Here's how the part is built. I have some questions about the finished solid (model axes, mm). A direction names the side the tool comes from. Coordinates: 2 decimals unless noted, no trailing zeros. Loops run counter-clockwise (first coordinate to the right, second up) from the corner with the lowest first, then second, coordinate; pieces in that order, holes last. Notation, with made-up numbers: (18, 41) -> (24, 41) arc R23 cw to (24, 58) -> close; hole circle Ø9 at (59.5, -37.75). An arc over 180 degrees is marked (long way). Answer as a JSON object with one key per item and string values. Group by question number.
1) I want a section at C-C (x = -20.5). Write out the boundary of the cut face in (y, z) (3 decimals), then the cut area to 3 significant figures.
2) I want a section at A-A (x = 0). Count the separate pieces of the cut face and the enclosed holes in it, then the cut area to 3 significant figures.
3) I need wall thicknesses on probe 1 along Y at (x, z) = (7.5, 11) (3 decimals); probe 2 along X at (y, z) = (-8, 16.5) (3 decimals); probe 3 along Z at (x, y) = (-11, -1.5). Which ranges of each line are inside material? Lowest first, please. Write a range as [from, to].
4) Which directions (+Z, -Z, +X, -X, +Y, -Y) give clear straight access to the entire face, cutting with the end or side of a thin tool? Please do faces 5 (the flat face through (-7, 6.096, 10)), 6 (the cylindrical face through (3.714, 8.478, 12.804)), 7 (the flat face through (-1, -6.223, 83)).
5) I'm going to push flat-ended pins straight in: pin 1 (4 mm diameter, centred on x = 5.14, z = 14.67, fed in from +Y); pin 2 (6 mm diameter, centred on x = -6.5, y = 0, fed in from -Z); pin 3 (1 mm diameter, centred on y = 5, z = 20.5, fed in from -X); pin 4 (4 mm diameter, centred on y = -4.5, z = 31, fed in from -X). Where does each tip first touch, or does it pass through?
6) If we mould it in two halves opening along X, with no side actions, what happens to faces 1 (the cylindrical face through (0.103, 8.541, 77.028)), 2 (the cylindrical face through (0.87, -8.54, 88.86)), 3 (the flat face through (9.525, 0, 39)), 4 (the flat face through (-7, -6.096, 10))? For each: +X half, -X half, draft (parallel to the pull), parting line (faces both ways), or undercut.
7) I want a section at D-D (y = 0). Write out the boundary of the cut face in (x, z) (3 decimals), then the cut area to 3 significant figures.
8) I want a section at B-B (z = 70). Write out the boundary of the cut face in (x, y) (3 decimals), then the cut area to 3 significant figures.
```python
from build123d import *

# Parameters (mm, degrees)
SKETCH1_W                    = 19.05
SKETCH1_H                    = 21.59
BOSS_EXTRUDE1_DEPTH          = 88.9
CUT_EXTRUDE_THIN1_DEPTH      = 92.978604713
CUT_EXTRUDE_THIN1_DEPTH_BACK = 88.9
SKETCH4_R                    = 2.3495
CUT_EXTRUDE1_DEPTH           = 92.978604713
BOSS_EXTRUDE2_START          = -21.59
SKETCH5_R                    = 2.3495
BOSS_EXTRUDE2_DEPTH          = 21.59
SKETCH6_W                    = 38.1
SKETCH6_H                    = 12.192
CUT_EXTRUDE2_DEPTH           = 96.446647008


with BuildPart() as part:
    # Sketch1 → Boss-Extrude1 (new body)
    with BuildSketch(Plane.XY):
        Rectangle(SKETCH1_W, SKETCH1_H)
    extrude(amount=BOSS_EXTRUDE1_DEPTH)

    # Sketch3 → Cut-Extrude-Thin1 (cut, two sides: drawn at the far end of the back side and taken through both)
    with BuildSketch(Plane(origin=(0, 10.795, 0), x_dir=(1, 0, 0), z_dir=(0, 1, 0)).offset(-CUT_EXTRUDE_THIN1_DEPTH_BACK)):
        with BuildLine():
            ThreePointArc((-9.525, -79.375), (0, -88.9), (9.525, -79.375))
            Line((9.525, -79.375), (34.925, -79.375))
            ThreePointArc((34.925, -79.375), (0, -114.3), (-34.925, -79.375))
            Line((-34.925, -79.375), (-9.525, -79.375))
        make_face()
    extrude(amount=CUT_EXTRUDE_THIN1_DEPTH + CUT_EXTRUDE_THIN1_DEPTH_BACK, mode=Mode.SUBTRACT)

    # Sketch4 → Cut-Extrude1 (cut, through all)
    with BuildSketch(Plane(origin=(0, 10.795, 0), x_dir=(1, 0, 0), z_dir=(0, 1, 0))):
        with Locations(Location((0, -79.375, 0), (0, 0, 270))):
            Circle(SKETCH4_R)
        with Locations(Location((5.1435, -14.6685, 0), (0, 0, 270))):
            Circle(SKETCH4_R)
        with Locations(Location((-5.1435, -4.3815, 0), (0, 0, 270))):
            Circle(SKETCH4_R)
    extrude(amount=-CUT_EXTRUDE1_DEPTH, mode=Mode.SUBTRACT)

    # Sketch5 → Boss-Extrude2 (add)
    with BuildSketch(Plane(origin=(0, 10.795, 0), x_dir=(1, 0, 0), z_dir=(0, 1, 0)).offset(BOSS_EXTRUDE2_START)):
        with BuildLine():
            Line((-9.525, -79.375), (-9.525, 0))
            Line((-9.525, 0), (-23.495, 0))
            Line((-23.495, 0), (-23.495, -19.05))
            Line((-23.495, -19.05), (-9.287597736, -81.488327539))
            ThreePointArc((-9.287597736, -81.488327539), (-9.465463365, -80.438310059), (-9.525, -79.375))
        make_face()
        with Locations(Location((-16.51, -9.525, 0), (0, 0, 270))):
            Circle(SKETCH5_R, mode=Mode.SUBTRACT)
    extrude(amount=BOSS_EXTRUDE2_DEPTH)

    # Sketch6 → Cut-Extrude2 (cut, through all)
    with BuildSketch(Plane(origin=(9.525, 0, 0), x_dir=(0, 0, -1), z_dir=(1, 0, 0))):
        Rectangle(SKETCH6_W, SKETCH6_H)
        with BuildLine():
            Line((-92.075, -6.223), (-72.898, -6.223))
            ThreePointArc((-72.898, -6.223), (-66.675, 0), (-72.898, 6.223))
            Line((-72.898, 6.223), (-92.075, 6.223))
            Line((-92.075, 6.223), (-92.075, -6.223))
        make_face()
    extrude(amount=-CUT_EXTRUDE2_DEPTH, mode=Mode.SUBTRACT)


solid = part.part
```
Determined:
{
 "1": {"outline": "(-10.795, 0) -> (-6.096, 0) -> (-6.096, 19.05) -> (6.096, 19.05) -> (6.096, 0) -> (10.795, 0) -> (10.795, 32.212) -> (-10.795, 32.212) -> close", "area": "463 mm^2"},
 "2": {"separate pieces": "3", "enclosed holes": "0", "area": "1,380 mm^2"},
 "3": {"probe 1": "[-10.795, -6.096], [6.096, 10.795]", "probe 2": "[-23.495, 3.672], [6.615, 9.525]", "probe 3": "[19.05, 66.86]"},
 "4": {"face 5": "-Z, +X, -X", "face 6": "+Y, -Y", "face 7": "+Z, +X, -X"},
 "5": {"pin 1": "through", "pin 2": "z = 19.05", "pin 3": "x = -23.28", "pin 4": "x = -21.23"},
 "6": {"face 1": "undercut", "face 2": "parting line", "face 3": "+X half", "face 4": "draft"},
 "7": {"outline": "(-23.495, 19.05) -> (9.525, 19.05) -> (9.525, 66.675) -> (-12.658, 66.675) -> close", "area": "1,310 mm^2"},
 "8": {"outline": "(-11.902, -10.795) -> (9.525, -10.795) -> (9.525, -5.507) -> (-11.902, -5.507) -> close; (-11.902, 5.507) -> (9.525, 5.507) -> (9.525, 10.795) -> (-11.902, 10.795) -> close", "area": "227 mm^2"}
}
